from build123d import *

# Parameters (mm, degrees)
F0_W          = 25
F0_H          = 30
F1_DEPTH      = 4
F2_R          = 1.675
F3_DEPTH      = 25
F4_W          = 25
F4_H          = 11
F5_DEPTH      = 13
F7_DEPTH      = 6
F8_R          = 8
F9_DEPTH      = 6
F2_R_2        = 3
F10_DEPTH     = 2
F11_W         = 11
F11_H         = 17
F12_DEPTH     = 2
F13_R         = 5
F14_W         = 11
F14_H         = 17
F15_DEPTH     = 2
F16_DEPTH     = 2
F17_R         = 1.45
F18_DEPTH     = 25
F19_T1_DEPTH  = 42
F19_T6_DEPTH  = 42
F19_T11_DEPTH = 42
F19_T16_DEPTH = 42
F19_T21_DEPTH = 42
F20_DEPTH     = 25


# Not quite as in the source:
# - a fillet or chamfer that OpenCascade refuses, or shapes differently, is made with other operations: its cross-section is extruded or revolved along the edge and cut away or added


with BuildPart() as f1:
    # F0 (on Top) → F1 (new body)
    with BuildSketch(Plane.XY):
        with Locations((12.5, 15)):
            Rectangle(F0_W, F0_H)
    extrude(amount=F1_DEPTH)

    # F2 (on face) → F3 (cut)
    with BuildSketch(Plane.XY.offset(4)):
        with BuildLine():
            ThreePointArc((3.325, 18.5605346784), (5, 16.8855346784), (6.675, 18.5605346784))
            ThreePointArc((6.675, 18.5605346784), (5, 20.2355346784), (3.325, 18.5605346784))
        make_face()
        with Locations((20, 18.5605346784)):
            Circle(F2_R)
        with Locations((20, 3.5605346784)):
            Circle(F2_R)
        with Locations((5, 3.5605346784)):
            Circle(F2_R)
    extrude(amount=-F3_DEPTH, mode=Mode.SUBTRACT)

    # F4 (on face) → F5 (join)
    with BuildSketch(Plane.XY.offset(4)):
        with Locations((12.5, 24.5)):
            Rectangle(F4_W, F4_H)
    extrude(amount=F5_DEPTH)

    # F6 (on face) → F7 (cut)
    with BuildSketch(Plane(origin=(0, 30, 0), x_dir=(-1, 0, 0), z_dir=(0, 1, 0))):
        with BuildLine():
            ThreePointArc((-18.5, 17), (-12.5, 11), (-6.5, 17))
            Line((-6.5, 17), (-18.5, 17))
        make_face()
    extrude(amount=-F7_DEPTH, mode=Mode.SUBTRACT)

    # F8 (on face) → F9 (cut)
    with BuildSketch(Plane.XZ.offset(-19)):
        with Locations((12.5, 17)):
            Circle(F8_R)
    extrude(amount=-F9_DEPTH, mode=Mode.SUBTRACT)

    # F2 (on face) → F10 (cut)
    with BuildSketch(Plane.XY.offset(4)):
        with BuildLine():
            ThreePointArc((8, 18.5605346784), (5, 21.5605346784), (2, 18.5605346784))
            ThreePointArc((2, 18.5605346784), (5, 15.5605346784), (8, 18.5605346784))
        make_face()
        with BuildLine():
            ThreePointArc((3.325, 18.5605346784), (5, 20.2355346784), (6.675, 18.5605346784))
            ThreePointArc((6.675, 18.5605346784), (5, 16.8855346784), (3.325, 18.5605346784))
        make_face(mode=Mode.SUBTRACT)
        with Locations((20, 18.5605346784)):
            Circle(F2_R_2)
        with Locations((20, 18.5605346784)):
            Circle(F2_R, mode=Mode.SUBTRACT)
        with Locations((20, 3.5605346784)):
            Circle(F2_R_2)
        with Locations((20, 3.5605346784)):
            Circle(F2_R, mode=Mode.SUBTRACT)
        with Locations((5, 3.5605346784)):
            Circle(F2_R_2)
        with Locations((5, 3.5605346784)):
            Circle(F2_R, mode=Mode.SUBTRACT)
    extrude(amount=-F10_DEPTH, mode=Mode.SUBTRACT)

    # F11 (on face) → F12 (join)
    with BuildSketch(Plane(origin=(0, 0, 0), x_dir=(0, -1, 0), z_dir=(-1, 0, 0))):
        with Locations((-24.5, 8.5)):
            Rectangle(F11_W, F11_H)
    extrude(amount=F12_DEPTH)

    # F13
    f13_edges = [f1.edges().sort_by_distance(p)[0] for p in [
        (0, 0, 2),
        (25, 0, 2),
    ]]
    fillet(f13_edges, radius=F13_R)

    # F14 (on face) → F15 (join)
    with BuildSketch(Plane.YZ.offset(25)):
        with Locations((24.5, 8.5)):
            Rectangle(F14_W, F14_H)
    extrude(amount=F15_DEPTH)

    # F14 (on face) → F16 (join)
    with BuildSketch(Plane.YZ.offset(25)):
        with Locations((24.5, 8.5)):
            Rectangle(F14_W, F14_H)
    extrude(amount=F16_DEPTH)

    # F17 (on face) → F18 (cut)
    with BuildSketch(Plane.XY.offset(17)):
        with Locations((0.45, 25.55)):
            Circle(F17_R)
        with Locations((24.55, 25.55)):
            Circle(F17_R)
    extrude(amount=-F18_DEPTH, mode=Mode.SUBTRACT)

    # F19: fillet of radius 5 on 4 edges, made by hand

    # F19_s2 → F19_t1 (cut)
    with BuildSketch(Plane.XY.offset(-12.5)):
        with BuildLine():
            ThreePointArc((-2, 25), (-0.5355339059, 28.5355339059), (3, 30))
            Line((3, 30), (-2, 30))
            Line((-2, 30), (-2, 25))
        make_face()
        with BuildLine():
            ThreePointArc((22, 30), (25.5355339059, 28.5355339059), (27, 25))
            Line((27, 25), (27, 30))
            Line((27, 30), (22, 30))
        make_face()
    extrude(amount=F19_T1_DEPTH, mode=Mode.SUBTRACT)


with BuildPart() as f19_tool4:
    # F19_s5 → F19_t6 (new body)
    with BuildSketch(Plane.XY.offset(-12.5)):
        with BuildLine():
            ThreePointArc((3, 19), (-0.5355339059, 20.4644660941), (-2, 24))
            Line((-2, 24), (-2, 19))
            Line((-2, 19), (3, 19))
        make_face()
    extrude(amount=F19_T6_DEPTH)

    split(bisect_by=Plane.YZ, keep=Keep.BOTTOM)


with BuildPart() as f1_1:
    add(f1.part)

    # F19_t3: cut F19_tool4
    add(f19_tool4.part, mode=Mode.SUBTRACT)


with BuildPart() as f19_tool9:
    # F19_s10 → F19_t11 (new body)
    with BuildSketch(Plane.XY.offset(-12.5)):
        with BuildLine():
            ThreePointArc((3, 19), (-0.5355339059, 20.4644660941), (-2, 24))
            Line((-2, 24), (-2, 19))
            Line((-2, 19), (3, 19))
        make_face()
    extrude(amount=F19_T11_DEPTH)

    split(bisect_by=Plane.XY.offset(4), keep=Keep.TOP)


with BuildPart() as f1_2:
    add(f1_1.part)

    # F19_t8: cut F19_tool9
    add(f19_tool9.part, mode=Mode.SUBTRACT)


with BuildPart() as f19_tool14:
    # F19_s15 → F19_t16 (new body)
    with BuildSketch(Plane.XY.offset(29.5)):
        with BuildLine():
            ThreePointArc((22, 19), (25.5355339059, 20.4644660941), (27, 24))
            Line((27, 24), (27, 19))
            Line((27, 19), (22, 19))
        make_face()
    extrude(amount=-F19_T16_DEPTH)

    split(bisect_by=Plane.XY.offset(4), keep=Keep.TOP)


with BuildPart() as f1_3:
    add(f1_2.part)

    # F19_t13: cut F19_tool14
    add(f19_tool14.part, mode=Mode.SUBTRACT)


with BuildPart() as f19_tool19:
    # F19_s20 → F19_t21 (new body)
    with BuildSketch(Plane.XY.offset(29.5)):
        with BuildLine():
            ThreePointArc((22, 19), (25.5355339059, 20.4644660941), (27, 24))
            Line((27, 24), (27, 19))
            Line((27, 19), (22, 19))
        make_face()
    extrude(amount=-F19_T21_DEPTH)

    split(bisect_by=Plane.YZ.offset(25), keep=Keep.TOP)


with BuildPart() as f1_4:
    add(f1_3.part)

    # F19_t18: cut F19_tool19
    add(f19_tool19.part, mode=Mode.SUBTRACT)

    # F2 (on face) → F20 (cut)
    with BuildSketch(Plane.XY.offset(4)):
        with BuildLine():
            ThreePointArc((8, 18.5605346784), (5, 21.5605346784), (2, 18.5605346784))
            ThreePointArc((2, 18.5605346784), (5, 15.5605346784), (8, 18.5605346784))
        make_face()
        with BuildLine():
            ThreePointArc((3.325, 18.5605346784), (5, 20.2355346784), (6.675, 18.5605346784))
            ThreePointArc((6.675, 18.5605346784), (5, 16.8855346784), (3.325, 18.5605346784))
        make_face(mode=Mode.SUBTRACT)
        with Locations((20, 18.5605346784)):
            Circle(F2_R_2)
        with Locations((20, 18.5605346784)):
            Circle(F2_R, mode=Mode.SUBTRACT)
        with BuildLine():
            ThreePointArc((3.325, 18.5605346784), (5, 16.8855346784), (6.675, 18.5605346784))
            ThreePointArc((6.675, 18.5605346784), (5, 20.2355346784), (3.325, 18.5605346784))
        make_face()
        with Locations((20, 18.5605346784)):
            Circle(F2_R)
    extrude(amount=F20_DEPTH, mode=Mode.SUBTRACT)


solid = f1_4.part
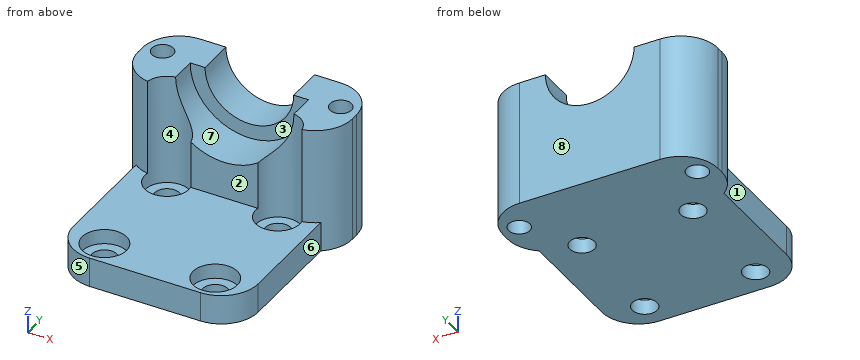
CAD build for the part. Positions are in the model's coordinates, mm. Face numbers are marked on the shaded views. A direction names the side the tool comes from. Give positions to 0.01 mm unless a question says otherwise; leave off trailing zeros. Loops run counter-clockwise (first coordinate to the right, second up) from the corner with the lowest first, then second, coordinate; pieces in that order, holes last. Notation, with made-up numbers: M 79,-4 L 83,-4 A13 ccw 83,0 Z; hole C 75,1.25 d4. An arc over 180 degrees is marked long. Write each question's results on one line, items separated by ' | '.
Q1. Flat gauge pins, fed straight in: P1, Ø3, axis at x = 20, y = 3.56, coming from the -Z side; P2, Ø10, axis at x = 15.5, z = 15, coming from the -Y side; P3, Ø3, axis at x = 19.5, y = 12, coming from the +Z side; P4, Ø2, axis at y = 13.5, z = 1.5, coming from the -X side. Where does each tip first touch, or does it go through?
Geometry check:
P1: passes through | P2: stops at y = 19 | P3: stops at z = 4 | P4: stops at x = 0
Q2. Mould opens along X. For the marked faces 5, 6, 7 and 8 say: pulls with the +X half, pulls with the -X half, needs draft (parallel to the pull), parting line crosses it, or undercut.
Geometry check:
face 5: pulls with the -X half | face 6: pulls with the +X half | face 7: undercut | face 8: needs draft
Q3. Band-saw the part on A-A on z = 6.75. Write the cut outline in (x, y).
Geometry check:
outline: M -2,24 A5 ccw 2.05,19.09 A3 cw 7.97,19 L 17.03,19 A3 cw 22.95,19.09 A5 ccw 27,24 L 27,25 A5 ccw 22,30 L 3,30 A5 ccw -2,25 Z; hole C 0.45,25.55 d2.9; hole C 24.55,25.55 d2.9
Q4. Band-saw the part on D-D on x = 0.45. Write the cut outline in (y, z), and give its area (3 significant figures).
Geometry check:
outline: M 2.93,0 L 24.1,0 L 24.1,17 L 19.7,17 L 19.7,4 L 2.93,4 Z; M 27,0 L 29.3,0 L 29.3,17 L 27,17 Z | area: 181 mm²
Q5. Probe probe 1 along Y at (x, z) = (20, 0.6); probe 2 along X at (y, z) = (6, 3.5); probe 3 along X at (y, z) = (25, 4). List the from-to ranges inside material, lowest first.
Geometry check:
probe 1: y = 0 to 1.89, 5.24 to 16.89, 20.24 to 30 | probe 2: x = 0 to 3.25, 6.75 to 18.25, 21.75 to 25 | probe 3: x = -2 to -0.89, 1.79 to 23.21, 25.89 to 27
Q6. Band-saw the part on B-B on z = 15.5. Write the cut outline in (x, y), and give its area (3 significant figures).
Geometry check:
outline: M -2,24 A5 ccw 2.05,19.09 A3 cw 4.64,21.54 L 4.64,25 L 6.69,25 L 6.69,30 L 3,30 A5 ccw -2,25 Z; M 18.31,25 L 20.36,25 L 20.36,21.54 A3 cw 22.95,19.09 A5 ccw 27,24 L 27,25 A5 ccw 22,30 L 18.31,30 Z; hole C 0.45,25.55 d2.9; hole C 24.55,25.55 d2.9 | area: 122 mm²
Q7. Band-saw the part on C-C on y = 19.5. Write the cut outline in (x, z).
Geometry check:
outline: M 0,0 L 3.61,0 L 3.61,2 L 2.15,2 L 2.15,17 L 0.82,17 L 0.82,4 L 0,4 Z; M 6.39,0 L 18.61,0 L 18.61,2 L 17.15,2 L 17.15,10.49 A8 cw 7.85,10.49 L 7.85,2 L 6.39,2 Z; M 21.39,0 L 25,0 L 25,4 L 24.18,4 L 24.18,17 L 22.85,17 L 22.85,2 L 21.39,2 Z
Q8. Which spindle directions (+Z, -Z, +X, -X, +Y, -Y) get a long thin tool onto all of the face, cutting with end or side? Do the marked faces 1, 2, 3 and 4. Say none if no direction does.
Geometry check:
face 1: +Z, -Z, -X, -Y | face 2: +Z, +X, -X, -Y | face 3: +Z, -Y | face 4: +Z
